Read the model definition and answer for the solid it produces. Units are mm, in the model's axes. Face numbers are marked on the shaded views. Coordinates: 2 decimals unless noted, no trailing zeros. Write each loop counter-clockwise with the first axis right and the second up, starting at its lowest first coordinate (ties: lowest second). Pieces come first, ordered by that corner, then holes.
Item 1: Section C-C (z = 8.5) is taken. Give the vertices of the cut face in (x, y).
Item 2: Each of these flat-tipped pins is pushed along its axis until it touches: P1, Ø1.5, axis at x = 5.5, z = 3.5, coming from the +Y side; P2, Ø2, axis at x = -10, z = 2.5, coming from the -Y side; P3, Ø6, axis at y = 2, z = 8.5, coming from the +X side. Where does it stop, or does it pass through?
Item 3: Straight lines are drawn through the part: probe 1 along Y at (x, z) = (0, 8); probe 2 along Z at (x, y) = (-8, 9.5); probe 3 along X at (y, z) = (4, -2.5). For each, find the intervals that lie inside material, in ascending order.
Item 4: Section D-D (y = 6) is taken. Give the vertices of the cut face in (x, z).
Item 5: Section A-A (x = 0) is taken. Give the vertices of the cut face in (y, z), then the cut area to 3 significant figures.
Item 6: Determine the mould class of the marked faces 1, 2 and 3 for opening direction X: released by +X, released by -X, zero draft, split by the parting line, or undercut.
Autodesk Inventor part; units mm, degrees
ref_plane "YZ Plane" through (0, 0, 0) normal (1, 0, 0) x (0, 1, 0)
ref_plane "XZ Plane" through (0, 0, 0) normal (0, 1, 0) x (-1, 0, 0)
ref_plane "XY Plane" through (0, 0, 0) normal (0, 0, 1) x (1, 0, 0)
sketch "Skizze1" plane through (0, 0, 0) normal (0, 1, 0) x (-1, 0, 0)
  line L0 (0, 20) -> (12.5, 20)
  line L1 (12.5, 20) -> (12.5, 19)
  line L2 (12.5, 19) -> (10, 19)
  line L3 (10, 19) -> (10, -19)
  line L4 (10, -19) -> (12.5, -19)
  line L5 (12.5, -19) -> (12.5, -20)
  line L6 (12.5, -20) -> (0, -20)
  line L7 (0, 20) -> (0, -20)
  line L8 (15, 0) -> (-2.5, 0)
  line L9 (0, -28) -> (0, 28)
  point P0 (0, 0)
  dimension "d4" = 20
  dimension "d5" = 25
  dimension "d6" = 40
  dimension "d7" = 1
revolve "Umdrehung1" add sketch "Skizze1" angle 360 about axis through (0, 0, 20) along (0, 0, -1)
sketch "Skizze2" plane through (0, 0, 20) normal (0, 0, 1) x (1, 0, 0)
  circle A0 centre (0, 0) radius 12.5
  circle A1 centre (0, 0) radius 5.05
  dimension "d1" = 10.1
extrude "Extrusion1" cut sketch "Skizze2" against normal through all contours A1
properties part number "Seil_Rolle_Antrieb"
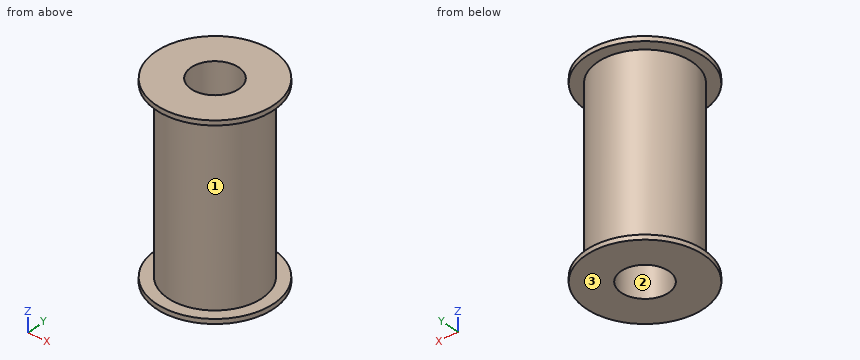
Established:
1. outline: circle Ø20 at (0, 0); hole circle Ø10.1 at (0, 0)
2. P1: stops at y = 8.8
2. P2: stops at y = -4.36
2. P3: stops at x = 10
3. probe 1: y = -10 to -5.05, 5.05 to 10
3. probe 2: z = -20 to -19, 19 to 20
3. probe 3: x = -9.17 to -3.08, 3.08 to 9.17
4. outline: (-10.97, -20) - (10.97, -20) - (10.97, -19) - (8, -19) - (8, 19) - (10.97, 19) - (10.97, 20) - (-10.97, 20) - (-10.97, 19) - (-8, 19) - (-8, -19) - (-10.97, -19) - close
5. outline: (-12.5, -20) - (-5.05, -20) - (-5.05, 20) - (-12.5, 20) - (-12.5, 19) - (-10, 19) - (-10, -19) - (-12.5, -19) - close; (5.05, -20) - (12.5, -20) - (12.5, -19) - (10, -19) - (10, 19) - (12.5, 19) - (12.5, 20) - (5.05, 20) - close
5. area: 406 mm2
6. face 1: split by the parting line
6. face 2: undercut
6. face 3: zero draft
